```python
from build123d import *

# Parameters (mm, degrees)
SKETCH1_W                   = 152.4
SKETCH1_H                   = 59.944
BOSS_EXTRUDE1_DEPTH         = 2.54
F_97_0_161_DIAMETER_HOLE1_D = 4.0894
F_97_0_75_DIAMETER_HOLE1_D  = 19.05


with BuildPart() as part:
    # Sketch1 → Boss-Extrude1 (new body)
    with BuildSketch(Plane(origin=(0, 0, 0), x_dir=(1, 0, 0), z_dir=(0, 1, 0))):
        with Locations((-76.2, 29.972)):
            Rectangle(SKETCH1_W, SKETCH1_H)
    extrude(amount=BOSS_EXTRUDE1_DEPTH)

    # #97 (0.161) Diameter Hole1 (through all)
    with Locations(Plane(origin=(0, 2.54, 0), x_dir=(1, 0, 0), z_dir=(0, 1, 0))):
        with Locations((-144.907, 47.879), (-127, 55.372), (-109.093, 47.879), (-109.093, 12.065), (-127, 4.572), (-144.907, 12.065)):
            Hole(F_97_0_161_DIAMETER_HOLE1_D / 2)

    # #97 (0.75) Diameter Hole1 (through all)
    with Locations(Plane(origin=(0, 2.54, 0), x_dir=(1, 0, 0), z_dir=(0, 1, 0))):
        with Locations((-127, 29.972)):
            Hole(F_97_0_75_DIAMETER_HOLE1_D / 2)


solid = part.part
```
CAD build for the part. Positions are in the model's coordinates, mm. Round coordinates to 2 decimals unless told otherwise and drop trailing zeros. Write each loop counter-clockwise with the first axis right and the second up, starting at its lowest first coordinate (ties: lowest second). Pieces come first, ordered by that corner, then holes. Notation, with made-up numbers: (-40, 81) - (-29, 81) arc R15 ccw to (-29, 90) - close; hole circle Ø2 at (71, 48). An arc over 180 degrees is marked (long way). Return JSON: item names as keys, results as strings. Group by question number.
Item 1: Flat gauge pin, fed straight in: pin 1 Ø12 at (x, z) = (-129, -47.5) entering from -Y. Where does the tip first touch, or does it go through?
Item 2: Band-saw the part on C-C on z = -25.5. List the corners of the cut face in (x, y).
Item 3: Probe probe 1 along Z at (x, y) = (-127, 1.2); probe 2 along X at (y, z) = (2.45, -49); probe 3 along X at (y, z) = (2.3, -11). List the from-to ranges inside material, lowest first.
Item 4: Band-saw the part on B-B on y = 1.65. List the corners of the cut face in (x, z) (3 decimals), plus the area to 3 significant figures.
Item 5: Band-saw the part on A-A on x = -127. List the corners of the cut face in (y, z).
Resolved:
{
 "1": {"pin 1": "stops at y = 0"},
 "2": {"outline": "(-152.4, 0) - (-135.41, 0) - (-135.41, 2.54) - (-152.4, 2.54) - close; (-118.59, 0) - (0, 0) - (0, 2.54) - (-118.59, 2.54) - close"},
 "3": {"probe 1": "z = -59.94 to -57.42, -53.33 to -39.5, -20.45 to -6.62, -2.53 to 0", "probe 2": "x = -152.4 to -146.62, -143.2 to -110.8, -107.38 to 0", "probe 3": "x = -152.4 to -146.65, -143.16 to -110.84, -107.35 to 0"},
 "4": {"outline": "(-152.4, -59.944) - (0, -59.944) - (0, 0) - (-152.4, 0) - close; hole circle Ø4.089 at (-144.907, -47.879); hole circle Ø4.089 at (-144.907, -12.065); hole circle Ø19.05 at (-127, -29.972); hole circle Ø4.089 at (-127, -55.372); hole circle Ø4.089 at (-127, -4.572); hole circle Ø4.089 at (-109.093, -47.879); hole circle Ø4.089 at (-109.093, -12.065)", "area": "8,770 mm²"},
 "5": {"outline": "(0, -59.94) - (2.54, -59.94) - (2.54, -57.42) - (0, -57.42) - close; (0, -53.33) - (2.54, -53.33) - (2.54, -39.5) - (0, -39.5) - close; (0, -20.45) - (2.54, -20.45) - (2.54, -6.62) - (0, -6.62) - close; (0, -2.53) - (2.54, -2.53) - (2.54, 0) - (0, 0) - close"}
}
